from build123d import *

# Parameters (mm, degrees)
BOSS_EXTRUDE1_DEPTH     = 20
CUT_EXTRUDE1_DEPTH      = 35.59205111
CUT_EXTRUDE1_DEPTH_BACK = 35.59205111
SKETCH4_R               = 2
BOSS_EXTRUDE2_START     = 20
BOSS_EXTRUDE2_DEPTH     = 5


with BuildPart() as part:
    # Sketch1 → Boss-Extrude1 (new body)
    with BuildSketch(Plane(origin=(0, 0, 0), x_dir=(1, 0, 0), z_dir=(0, 1, 0))):
        Polygon((15.1, -14), (15.1, 14), (2, 14), (2, 25), (0, 25), (0, 12), (13.1, 12), (13.1, -12), (0, -12), (0, -25), (2, -25), (2, -14), align=None)
    extrude(amount=BOSS_EXTRUDE1_DEPTH)

    # Sketch4 → Cut-Extrude1 (cut, two sides: drawn at the far end of the back side and taken through both)
    with BuildSketch(Plane(origin=(2, 0, 0), x_dir=(0, 0, -1), z_dir=(1, 0, 0)).offset(-CUT_EXTRUDE1_DEPTH_BACK)):
        with Locations((-19.5, 8)):
            Circle(SKETCH4_R)
        with Locations(Location((19.5, 8, 0), (0, 0, 180))):
            Circle(SKETCH4_R)
    extrude(amount=CUT_EXTRUDE1_DEPTH + CUT_EXTRUDE1_DEPTH_BACK, mode=Mode.SUBTRACT)

    # Sketch1<31> → Boss-Extrude2 (add)
    with BuildSketch(Plane(origin=(0, 0, 0), x_dir=(1, 0, 0), z_dir=(0, 1, 0)).offset(BOSS_EXTRUDE2_START)):
        with BuildLine():
            Line((15.1, -25), (15.1, -14))
            Line((15.1, -14), (6.55, -14))
            Line((6.55, -14), (6.55, -19))
            ThreePointArc((6.55, -19), (7.964213562, -19.585786438), (8.55, -21))
            ThreePointArc((8.55, -21), (7.964213562, -22.414213562), (6.55, -23))
            Line((6.55, -23), (6.55, -25))
            Line((6.55, -25), (15.1, -25))
        make_face()
        with BuildLine():
            Line((6.55, -19), (6.55, -14))
            Line((6.55, -14), (2, -14))
            Line((2, -14), (2, -25))
            Line((2, -25), (6.55, -25))
            Line((6.55, -25), (6.55, -23))
            ThreePointArc((6.55, -23), (4.55, -21), (6.55, -19))
        make_face()
        with BuildLine():
            Line((6.55, 14), (15.1, 14))
            Line((15.1, 14), (15.1, 25))
            Line((15.1, 25), (6.55, 25))
            Line((6.55, 25), (6.55, 23))
            ThreePointArc((6.55, 23), (7.964213562, 22.414213562), (8.55, 21))
            ThreePointArc((8.55, 21), (7.964213562, 19.585786438), (6.55, 19))
            Line((6.55, 19), (6.55, 14))
        make_face()
        with BuildLine():
            Line((2, 14), (6.55, 14))
            Line((6.55, 14), (6.55, 19))
            ThreePointArc((6.55, 19), (4.55, 21), (6.55, 23))
            Line((6.55, 23), (6.55, 25))
            Line((6.55, 25), (2, 25))
            Line((2, 25), (2, 14))
        make_face()
    extrude(amount=-BOSS_EXTRUDE2_DEPTH)


solid = part.part
For this review, take the finished solid that the model builds, in its own axes (mm). A direction names the side the tool comes from. Round coordinates to 2 decimals unless told otherwise and drop trailing zeros. Order: outer loops, then holes, each group sorted by start corner. A loop starts at its lowest first (then second) coordinate and runs counter-clockwise, first axis right, second up. Notation, with made-up numbers: M 78.5,2 L 84.5,2 A26 ccw 84.5,18 Z; hole C 34,34 d6. An arc over 180 degrees is marked long. Use a Markdown table: item, result. Add a question column.
Item 1: Tool access review of faces 5 (the flat face through (2, 5.7, -19.4)), 6 (the flat face through (8, 15, 19)), 7 (the flat face through (7, 10, 12)): name each direction out of +Z, -Z, +X, -X, +Y, -Y from which nothing blocks a thin tool from reaching the whole face with its end or side.
Item 2: Add section A-A, the plane y = 8. Give the boundary of the cut face in (x, z).
Item 3: Add section D-D, the plane z = 11. Give the boundary of the cut face in (x, y).
Item 4: To check wall thickness, follow line 1 along Y through (x, z) = (1.55, -19.5); line 2 along Z through (x, y) = (10.25, 14); line 3 along X through (y, z) = (14.75, -21). State the ranges of each line that lie inside material, in increasing order.
Item 5: Insertion check: pin 1 (3 mm diameter, centred on y = 8, z = 19.5, fed in from -X); pin 2 (6.5 mm diameter, centred on x = 11.5, y = 5.5, fed in from -Z); pin 3 (3.5 mm diameter, centred on x = 9.5, z = -21, fed in from -Y); pin 4 (9 mm diameter, centred on y = 5.5, z = -20, fed in from +X). Each pin has a flat end and moves straight along its axis. Give the tip position at first contact, or say it passes through.
Item 6: Add section C-C, the plane z = 17. Give the boundary of the cut face in (x, y), then the cut area to 4 significant figures.
Item 7: Add section B-B, the plane y = 10.75. Give the boundary of the cut face in (x, z).
Item 8: Mouldability with a two-part tool opening along Z and no side actions: class faces 1 (the flat face through (14, 0, 0)), 2 (the flat face through (13.1, 10, 0)), 3 (the flat face through (8, 7, 14)), 4 (the flat face through (6, 10, -12)) as released by +Z, released by -Z, zero draft, split by the parting line, or undercut.
Geometry results:
| question | item | result |
|---|---|---|
| 1 | face 5 | -Z, +X, -Y |
| 1 | face 6 | +Z, +X, -Y |
| 1 | face 7 | -X, +Y, -Y |
| 2 | outline | M 0,-25 L 2,-25 L 2,-21.5 L 0,-21.5 Z; M 0,-17.5 L 2,-17.5 L 2,-14 L 15.1,-14 L 15.1,14 L 2,14 L 2,17.5 L 0,17.5 L 0,12 L 13.1,12 L 13.1,-12 L 0,-12 Z; M 0,21.5 L 2,21.5 L 2,25 L 0,25 Z |
| 3 | outline | M 13.1,0 L 15.1,0 L 15.1,20 L 13.1,20 Z |
| 4 | line 1 | y = 0 to 6, 10 to 20 |
| 4 | line 2 | z = -14 to -12, 12 to 14 |
| 4 | line 3 | x = 0 to 2 |
| 5 | pin 1 | passes through |
| 5 | pin 2 | stops at z = -14 |
| 5 | pin 3 | stops at y = 15 |
| 5 | pin 4 | stops at x = 2 |
| 6 | outline | M 0,0 L 2,0 L 2,15 L 15.1,15 L 15.1,20 L 0,20 Z |
| 6 | area | 105.5 mm² |
| 7 | outline | M 0,-25 L 2,-25 L 2,-14 L 15.1,-14 L 15.1,14 L 2,14 L 2,25 L 0,25 L 0,12 L 13.1,12 L 13.1,-12 L 0,-12 Z |
| 8 | face 1 | zero draft |
| 8 | face 2 | undercut |
| 8 | face 3 | released by +Z |
| 8 | face 4 | undercut |
